Autodesk Inventor part; units mm, degrees
ref_plane "Work Plane2" through (-110.9217, -110.9217, -15) normal (0, 0, -1) x (0, 1, 0)
ref_plane "YZ Plane" through (0, 0, 0) normal (1, 0, 0) x (0, 1, 0)
ref_plane "XZ Plane" through (0, 0, 0) normal (0, 1, 0) x (-1, 0, 0)
ref_plane "Work Plane1" through (-132.9045, 0, 0) normal (0, 0, 1) x (1, 0, 0)
ref_plane "Work Plane2" through (-110.9217, -110.9217, -15) normal (0, 0, -1) x (0, 1, 0)
sketch "Sketch1" plane through (-132.9045, 0, 0) normal (0, 0, 1) x (1, 0, 0)
  arc A0 (116.9045, 94.6573) -> (116.9045, -94.6573) centre (132.9045, 0) ccw
  arc A1 (116.9045, -94.6573) -> (131.4538, -104) centre (131.4538, -88) ccw
  line L0 (131.4538, -104) -> (134.3553, -104)
  arc A2 (134.3553, -104) -> (148.9045, -94.6573) centre (134.3553, -88) ccw
  arc A3 (148.9045, -94.6573) -> (206.8801, -61.185) centre (132.9045, 0) ccw
  arc A4 (206.8801, -61.185) -> (222.2458, -53.2564) centre (208.3894, -45.2564) ccw
  line L1 (222.2458, -53.2564) -> (223.6965, -50.7436)
  arc A5 (223.6965, -50.7436) -> (222.8801, -33.4722) centre (209.8401, -42.7436) ccw
  arc A6 (222.8801, -33.4722) -> (222.8801, 33.4722) centre (132.9045, 0) ccw
  arc A7 (222.8801, 33.4722) -> (223.6965, 50.7436) centre (209.8401, 42.7436) ccw
  line L2 (223.6965, 50.7436) -> (222.2458, 53.2564)
  arc A8 (222.2458, 53.2564) -> (206.8801, 61.185) centre (208.3894, 45.2564) ccw
  arc A9 (206.8801, 61.185) -> (148.9045, 94.6573) centre (132.9045, 0) ccw
  arc A10 (148.9045, 94.6573) -> (134.3553, 104) centre (134.3553, 88) ccw
  line L3 (134.3553, 104) -> (131.4538, 104)
  arc A11 (131.4538, 104) -> (116.9045, 94.6573) centre (131.4538, 88) ccw
  circle A12 centre (132.9045, 0) radius 3.5
  circle A13 centre (132.9045, -100) radius 3
  circle A14 centre (63.6225, -40) radius 3.5
  circle A15 centre (132.9045, -80) radius 3.5
  circle A16 centre (202.1866, -40) radius 3.5
  circle A17 centre (202.1866, 40) radius 3.5
  circle A18 centre (132.9045, 80) radius 3.5
  circle A19 centre (63.6225, 40) radius 3.5
  circle A20 centre (219.5071, -50) radius 3
  circle A21 centre (219.5071, 50) radius 3
  circle A22 centre (132.9045, 100) radius 3
  line L4 (36.9045, 0) -> (36.9045, 30)
  line L5 (36.9045, 30) -> (41.7124, 30)
  line L6 (36.9045, 0) -> (36.9045, -30)
  line L7 (36.9045, -30) -> (41.7124, -30)
  line L8 (36.9045, 30) -> (-58.0955, 30)
  line L9 (-58.0955, 30) -> (-58.0955, -30)
  line L10 (-58.0955, -30) -> (36.9045, -30)
  line L11 (36.9045, -30) -> (36.9045, 30)
  circle A23 centre (48.0955, -16) radius 2.1
  circle A24 centre (48.0955, 16) radius 2.1
  point P0 (132.9045, 0)
  dimension "d0" = 30
  dimension "d1" = 30
  dimension "d2" = 95
  dimension "d3" = 60
extrude "Extrusion1" add sketch "Sketch1" against normal up to surface (15 mm away) contours A0 L4 L5 | L6 L10 L9 L8 L4 | A0 L7 L6
sketch "Sketch2" plane through (-91.1921, 30, -15) normal (0, 0, -1) x (-1, 0, 0)
  circle A0 centre (-91.1921, -30) radius 3.5
  arc A1 (-91.1921, 66) -> (-174.3305, 18) centre (-91.1921, -30) ccw
  circle A2 centre (-160.4741, 10) radius 16
  arc A3 (-174.3305, 18) -> (-174.3305, -78) centre (-91.1921, -30) ccw
  circle A4 centre (-160.4741, -70) radius 16
  arc A5 (-174.3305, -78) -> (-91.1921, -126) centre (-91.1921, -30) ccw
  circle A6 centre (-91.1921, -110) radius 16
  arc A7 (-91.1921, -126) -> (-8.0537, -78) centre (-91.1921, -30) ccw
  circle A8 centre (-21.9101, -70) radius 16
  arc A9 (-8.0537, -78) -> (-8.0537, 18) centre (-91.1921, -30) ccw
  circle A10 centre (-21.9101, 10) radius 16
  arc A11 (-8.0537, 18) -> (-91.1921, 66) centre (-91.1921, -30) ccw
  circle A12 centre (-91.1921, 50) radius 16
  line L0 (99.8079, 0) -> (99.8079, -60)
  line L1 (0, 0) -> (99.8079, 0)
  arc A13 (0, -60) -> (0, 0) centre (-91.1921, -30) ccw
  line L2 (99.8079, -60) -> (0, -60)
  circle A14 centre (-6.383, -14) radius 2.1
  line L3 (0, 0) -> (-16.383, -11.4715)
  line L4 (0, 0) -> (20, 0) construction
  line L5 (0, -60) -> (-16.383, -48.5285)
  line L6 (0, -60) -> (20, -60) construction
  line L7 (99.8079, -60) -> (0, -60)
  line L8 (-16.383, -48.5285) -> (-16.383, -11.4715)
  circle A15 centre (-6.383, -46) radius 2.1
  circle A16 centre (-6.383, -46) radius 2.1
  circle A17 centre (-6.383, -14) radius 2.1
  point P0 (-91.1921, -30)
  dimension "d6" = 4.2
  dimension "d7" = 14
  dimension "d8" = 20
  dimension "d9" = 145
  dimension "d10" = 20
  dimension "d11" = 145
  dimension "d12" = 10
  dimension "d13" = 14
  dimension "d14" = 10
extrude "Extrusion2" add sketch "Sketch2" along normal blind 8 contours L1 L0 L2 A9 | A9 L5 L8 L3
sketch "Sketch3" plane through (-91.1921, 30, -23) normal (0, 0, -1) x (-1, 0, 0)
  line L0 (38.3079, -51.5) -> (81.3079, -51.5)
  line L1 (81.3079, -51.5) -> (81.3079, -8.5)
  line L2 (81.3079, -8.5) -> (38.3079, -8.5)
  line L3 (38.3079, -8.5) -> (38.3079, -51.5)
  line L4 (38.3079, -51.5) -> (81.3079, -8.5) construction
  line L5 (81.3079, -51.5) -> (38.3079, -8.5) construction
  line L6 (99.8079, -60) -> (99.8079, 0)
  line L7 (99.8079, 0) -> (0, 0)
  line L8 (99.8079, -60) -> (0, -60)
  line L9 (99.8079, 0) -> (23.3079, 0)
  line L10 (23.3079, 0) -> (23.3079, -60)
  line L11 (23.3079, -60) -> (99.8079, -60)
  line L12 (99.8079, -60) -> (99.8079, 0)
  line L13 (28.3079, -55) -> (28.3079, -5)
  line L14 (28.3079, -5) -> (94.8079, -5)
  line L15 (94.8079, -5) -> (94.8079, -55)
  line L16 (94.8079, -55) -> (28.3079, -55)
  point P0 (-91.1921, -30)
  point P1 (59.8079, -30)
  point P2 (23.3079, 0)
  dimension "d17" = 43
  dimension "d18" = 43
  dimension "d26" = 30
  dimension "d29" = 40
  dimension "d30" = 15
  dimension "d31" = 5
extrude "Extrusion3" add sketch "Sketch3" along normal blind 24 contours L8 L10 L7 L6
sketch "Sketch4" plane through (-91.1921, 30, -47) normal (0, 0, -1) x (-1, 0, 0)
  circle A0 centre (41.8079, -14.5) radius 1.5
  circle A1 centre (41.8079, -45.5) radius 1.5
  circle A2 centre (72.8079, -14.5) radius 1.5
  circle A3 centre (72.8079, -45.5) radius 1.5
  circle A4 centre (57.3079, -30) radius 11
  line L0 (76.3079, -9) -> (78.3079, -11)
  line L1 (76.3079, -9) -> (38.3079, -9)
  line L2 (36.3079, -11) -> (38.3079, -9)
  line L3 (36.3079, -11) -> (36.3079, -49)
  line L4 (38.3079, -51) -> (36.3079, -49)
  line L5 (38.3079, -51) -> (76.3079, -51)
  line L6 (78.3079, -49) -> (76.3079, -51)
  line L7 (78.3079, -49) -> (78.3079, -11)
  line L8 (23.3079, -60) -> (99.8079, -60)
  line L9 (99.8079, -60) -> (99.8079, 0)
  line L10 (99.8079, 0) -> (23.3079, 0)
  line L11 (23.3079, 0) -> (23.3079, -60)
  line L12 (28.3079, -55) -> (28.3079, -5)
  line L13 (28.3079, -5) -> (94.8079, -5)
  line L14 (94.8079, -5) -> (94.8079, -55)
  line L15 (94.8079, -55) -> (28.3079, -55)
  point P0 (-91.1921, -30)
extrude "Extrusion4" cut sketch "Sketch4" against normal through all contours A1 | A2 | A3 | A4
sketch "Sketch5" plane through (-91.1921, 30, -23) normal (0, 0, -1) x (-1, 0, 0)
  circle A0 centre (41.8079, -45.5) radius 1.5
  circle A1 centre (57.3079, -30) radius 11
  circle A2 centre (72.8079, -45.5) radius 1.5
  circle A3 centre (72.8079, -14.5) radius 1.5
  line L0 (28.3079, -55) -> (94.8079, -55)
  line L1 (94.8079, -55) -> (94.8079, -5)
  line L2 (94.8079, -5) -> (28.3079, -5)
  line L3 (28.3079, -5) -> (28.3079, -55)
  point P0 (-91.1921, -30)
extrude "Extrusion5" cut sketch "Sketch5" against normal through all
sketch "Sketch6" plane through (-91.1921, 30, -47) normal (0, 0, -1) x (-1, 0, 0)
  line L0 (23.3079, -60) -> (99.8079, -60)
  line L1 (99.8079, -60) -> (99.8079, 0)
  line L2 (99.8079, 0) -> (23.3079, 0)
  line L3 (23.3079, 0) -> (23.3079, -60)
  line L4 (28.3079, -55) -> (28.3079, -5)
  line L5 (28.3079, -5) -> (94.8079, -5)
  line L6 (94.8079, -5) -> (94.8079, -55)
  line L7 (94.8079, -55) -> (28.3079, -55)
  circle A0 centre (41.8079, -14.5) radius 1.5
  circle A1 centre (72.8079, -14.5) radius 1.5
  circle A2 centre (72.8079, -45.5) radius 1.5
  circle A3 centre (41.8079, -45.5) radius 1.5
  circle A4 centre (41.8079, -14.5) radius 1.7
  circle A5 centre (72.8079, -14.5) radius 1.7
  circle A6 centre (72.8079, -45.5) radius 1.7
  circle A7 centre (41.8079, -45.5) radius 1.7
  line L8 (41.8079, -43.8) -> (72.8079, -43.8)
  line L9 (72.8079, -47.2) -> (41.8079, -47.2)
  line L10 (41.8079, -12.8) -> (72.8079, -12.8)
  line L11 (72.8079, -16.2) -> (41.8079, -16.2)
  line L12 (41.8079, -16.2) -> (28.3079, -16.2)
  line L13 (41.8079, -12.8) -> (28.3079, -12.8)
  line L14 (72.8079, -12.8) -> (94.8079, -12.8)
  line L15 (72.8079, -16.2) -> (94.8079, -16.2)
  line L16 (72.8079, -43.8) -> (94.8079, -43.8)
  line L17 (72.8079, -47.2) -> (94.8079, -47.2)
  line L18 (41.8079, -47.2) -> (28.3079, -47.2)
  line L19 (41.8079, -43.8) -> (28.3079, -43.8)
  circle A8 centre (57.3079, -30) radius 11
  circle A9 centre (57.3079, -30) radius 11.5
  line L20 (57.3079, -18.5) -> (28.3079, -18.5)
  line L21 (57.3079, -18.5) -> (94.8079, -18.5)
  line L22 (57.3079, -41.5) -> (94.8079, -41.5)
  line L23 (57.3079, -41.5) -> (28.3079, -41)
  point P0 (-91.1921, -30)
  point P1 (56.9115, -41.4932)
  dimension "d32" = 0.2
  dimension "d33" = 0.2
  dimension "d34" = 0.2
  dimension "d35" = 0.2
  dimension "d39" = 0.5
extrude "Extrusion6" add sketch "Sketch6" along normal blind 5 contours L3 L2 L1 L0 | L4 L18 L9 L17 L6 L7 | L4 L23 L22 L6 L16 L8 L19 | L4 L12 L11 L15 L6 L21 L20 | L4 L5 L6 L14 L10 L13
fillet "Fillet1" radius 3 7 edges at (-114.5, -30, -37.5) (-152.75, -30, -52) (-114.5, 0, -52) (-152.75, 30, -52) (-191, -30, -26) (-191, 0, -52) (-191, 30, -26)
sketch "Sketch7" plane through (-191, -27, 0) normal (-1, 0, 0) x (0, 0, 1)
  line L0 (0, 27) -> (-20, 27)
  line L1 (-20, 27) -> (-20, 17.9937)
  line L2 (-20, 17.9937) -> (0, 17.9937)
  line L3 (0, 17.9937) -> (0, 27)
  line L4 (0, 27) -> (-20, 27)
  line L5 (-20, 27) -> (-20, 35.9937)
  line L6 (-20, 35.9937) -> (0, 35.9937)
  line L7 (0, 35.9937) -> (0, 27)
  dimension "d41" = 20
  dimension "d42" = 18
extrude "Extrusion7" cut sketch "Sketch7" against normal up to surface (5 mm away)
properties part number "base-stepper-holder_3DPrint"
The listing builds one solid part. Answer for the finished solid, in the listing's coordinates (mm). A direction names the side the tool comes from. Give positions to 0.01 mm unless a question says otherwise; leave off trailing zeros. Order: outer loops, then holes, each group sorted by start corner. A loop starts at its lowest first (then second) coordinate and runs counter-clockwise, first axis right, second up. Notation, with made-up numbers: (-7.75, 12) - (11.25, 12) arc R19 ccw to (11.25, 28) - close; hole circle Ø3 at (-15.5, -23.5). An arc over 180 degrees is marked (long way). Answer as CSV lines item,"result".
Q1. A cutting plane is placed at D-D, the plane z = -43. Determine the outline of the cut face in (x, y), and give its area (3 significant figures).
Answer key:
outline,"(-191, -27) arc R3 ccw to (-188, -30) - (-117.5, -30) arc R3 ccw to (-114.5, -27) - (-114.5, 30) - (-188, 30) arc R3 ccw to (-191, 27) - close; hole (-186, -25) - (-119.5, -25) - (-119.5, 25) - (-186, 25) - close"
area,"1,260 mm^2"
Q2. Determine the mould class of faces 5 (the face through (-140, -30, -24)), 6 (the face through (-74.809, 0, -19)), 7 (the face through (-83.115, 24.345, -18.944)), 8 (the face through (-152, -13.8, -49)) for opening direction Y: pulls with the +Y half, pulls with the -Y half, needs draft (parallel to the pull), parting line crosses it, or undercut.
Answer key:
face 5,"pulls with the -Y half"
face 6,"needs draft"
face 7,"pulls with the +Y half"
face 8,"undercut"
Q3. Which of the six approach directions +Z, -Z, +X, -X, +Y, -Y give full straight-line access (tool end or side, diameter ignored) to faces 1 (the face through (-85, 0, -15)), 2 (the face through (-186, 0, -26)), 3 (the face through (-152, 17.2, -49)), 4 (the face through (-189, 0, -20))?
Answer key:
face 1,"+Z, +X"
face 2,"+Z"
face 3,"+Z, -Z"
face 4,"+Z, -X"
Q4. A cutting plane is placed at B-B, the plane y = 7.5. Determine the outline of the cut face in (x, z).
Answer key:
outline,"(-191, -49) arc R3 ccw to (-188, -52) - (-186, -52) - (-186, -20) - (-191, -20) - close; (-119.5, -52) - (-117.5, -52) arc R3 ccw to (-114.5, -49) - (-114.5, -23) - (-74.81, -23) - (-74.81, -15) - (-95.71, -15) - (-95.71, 0) - (-119.5, 0) - close"
Q5. Straight lines are drawn through the part: L1, parallel to X at y = 13.5, z = -25; L2, parallel to Y at x = -142, z = -34.5; L3, parallel to Y at x = -137, z = -47.5. For each, find the intervals that lie inside material, in ascending order.
Answer key:
L1,"x = -191 to -186, -119.5 to -114.5"
L2,"y = -30 to -25, 25 to 30"
L3,"y = -30 to -17.2, -13.8 to -11.3, 11.5 to 13.8, 17.2 to 30"
Q6. A cutting plane is placed at A-A, the plane x = -160.5. Determine the outline of the cut face in (y, z).
Answer key:
outline,"(-30, -49) arc R3 ccw to (-27, -52) - (-17.2, -52) - (-17.2, -47) - (-25, -47) - (-25, 0) - (-30, 0) - close; (-13.8, -52) - (-11.5, -52) - (-11.5, -47) - (-13.8, -47) - close; (11.5, -52) - (13.8, -52) - (13.8, -47) - (11.5, -47) - close; (17.2, -52) - (27, -52) arc R3 ccw to (30, -49) - (30, 0) - (25, 0) - (25, -47) - (17.2, -47) - close"
Q7. A cutting plane is placed at C-C, the plane z = -17. Determine the outline of the cut face in (x, y).
Answer key:
outline,"(-191, -27) arc R3 ccw to (-188, -30) - (-91.19, -30) - (-74.81, -18.53) - (-74.81, 18.53) - (-91.19, 30) - (-188, 30) arc R3 ccw to (-191, 27) - (-191, 8.99) - (-186, 8.99) - (-186, 25) - (-119.5, 25) - (-119.5, -25) - (-186, -25) - (-186, -9.01) - (-191, -9.01) - close; hole circle Ø4.2 at (-84.81, -16); hole circle Ø4.2 at (-84.81, 16)"
Q8. Each of these flat-tipped pins is pushed along its axis until it touches: pin 1 Ø1.5 at (x, z) = (-117, -23.5) entering from -Y; pin 2 Ø2 at (y, z) = (-5.5, -17.5) entering from -X; pin 3 Ø4 at (x, y) = (-144, -19) entering from +Z; pin 4 Ø3 at (y, z) = (1, -45) entering from +X. Where does it stop, or does it pass through?
Answer key:
pin 1,"stops at y = -30"
pin 2,"stops at x = -119.5"
pin 3,"stops at z = -47"
pin 4,"stops at x = -114.5"
